Answer from the drawing. Dimensions are ordinates in mm from the lowest x, y and z of the part. A direction names the side the tool comes from. Give positions to 0.01 mm unless a question says otherwise; leave off trailing zeros. Loops run counter-clockwise (first coordinate to the right, second up) from the corner with the lowest first, then second, coordinate; pieces in that order, holes last. Notation, with made-up numbers: (-21, 1.25) -> (15, 1.25) arc R20 cw to (15, 40.25) -> close; hole circle Ø10 at (48.25, 26.25). An arc over 180 degrees is marked (long way). Return JSON: item names as keys, results as strings. Group by question number.
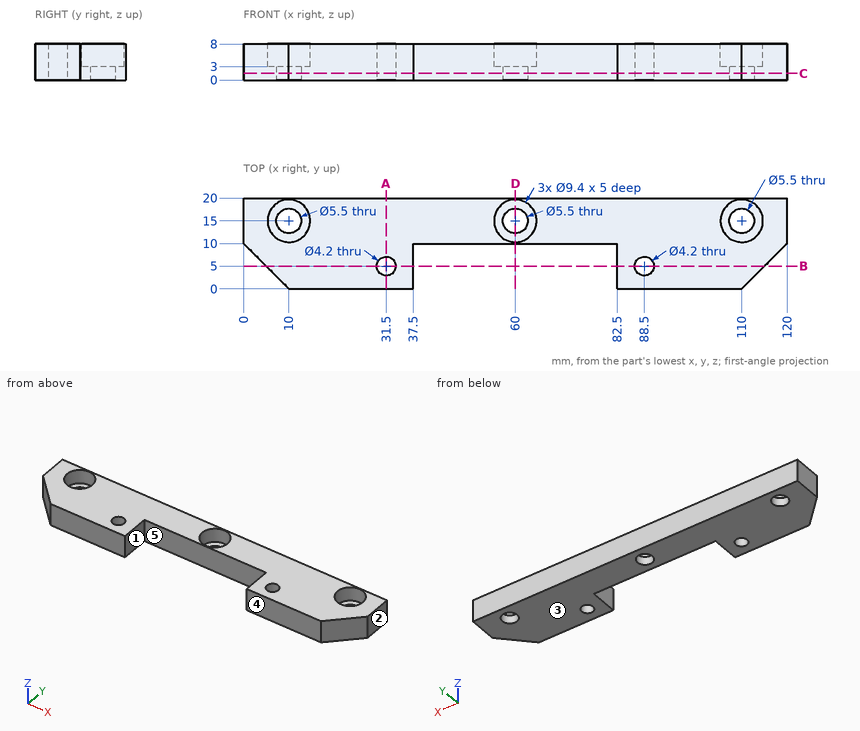
1. Section B-B on y = 5 is taken. Determine the outline of the cut face in (x, z), then the cut area to 3 significant figures.
2. Section C-C on z = 1.5 is taken. Determine the outline of the cut face in (x, y).
3. Section D-D on x = 60 is taken. Determine the outline of the cut face in (y, z), then the cut area to 3 significant figures.
4. Section A-A on x = 31.5 is taken. Determine the outline of the cut face in (y, z), then the cut area to 3 significant figures.
5. Straight lines are drawn through the part: line 1 (Y direction, x = 60, z = 2.2); line 2 (Y direction, x = 60, z = 6.55); line 3 (X direction, y = 6, z = 2.5). For each, find the intervals that lie inside material, in ascending order. Write a range as from..to.
6. Which of the six approach directions +Z, -Z, +X, -X, +Y, -Y give full straight-line access (tool end or side, diameter ignored) to the marked faces 4 and 5?
7. Flat-ended cylindrical pins translate along their axes: pin 1 Ø3 at (x, y) = (10, 14) entering from +Z; pin 2 Ø3 at (x, y) = (58, 16.5) entering from +Z; pin 3 Ø2.5 at (y, z) = (2.5, 4) entering from -X. Find the tip coordinate at first contact, or state that the pin passes through.
8. Determine the mould class of the marked faces 1, 2 and 3 for opening direction X: pulls with the +X half, pulls with the -X half, needs draft (parallel to the pull), parting line crosses it, or undercut.
Completed:
{
 "1": {"outline": "(5, 0) -> (29.4, 0) -> (29.4, 8) -> (5, 8) -> close; (33.6, 0) -> (37.5, 0) -> (37.5, 8) -> (33.6, 8) -> close; (82.5, 0) -> (86.4, 0) -> (86.4, 8) -> (82.5, 8) -> close; (90.6, 0) -> (115, 0) -> (115, 8) -> (90.6, 8) -> close", "area": "453 mm²"},
 "2": {"outline": "(0, 10) -> (10, 0) -> (37.5, 0) -> (37.5, 10) -> (82.5, 10) -> (82.5, 0) -> (110, 0) -> (120, 10) -> (120, 20) -> (0, 20) -> close; hole circle Ø5.5 at (10, 15); hole circle Ø4.2 at (31.5, 5); hole circle Ø5.5 at (60, 15); hole circle Ø4.2 at (88.5, 5); hole circle Ø5.5 at (110, 15)"},
 "3": {"outline": "(10, 0) -> (12.25, 0) -> (12.25, 3) -> (10.3, 3) -> (10.3, 8) -> (10, 8) -> close; (17.75, 0) -> (20, 0) -> (20, 8) -> (19.7, 8) -> (19.7, 3) -> (17.75, 3) -> close", "area": "16.5 mm²"},
 "4": {"outline": "(0, 0) -> (2.9, 0) -> (2.9, 8) -> (0, 8) -> close; (7.1, 0) -> (20, 0) -> (20, 8) -> (7.1, 8) -> close", "area": "126 mm²"},
 "5": {"line 1": "y = 10..12.25, 17.75..20", "line 2": "y = 10..10.3, 19.7..20", "line 3": "x = 4..29.65, 33.35..37.5, 82.5..86.65, 90.35..116"},
 "6": {"face 4": "+Z, -Z, +X, -X, -Y", "face 5": "+Z, -Z, -Y"},
 "7": {"pin 1": "passes through", "pin 2": "stops at z = 3", "pin 3": "stops at x = 6.25"},
 "8": {"face 1": "undercut", "face 2": "pulls with the +X half", "face 3": "needs draft"}
}
